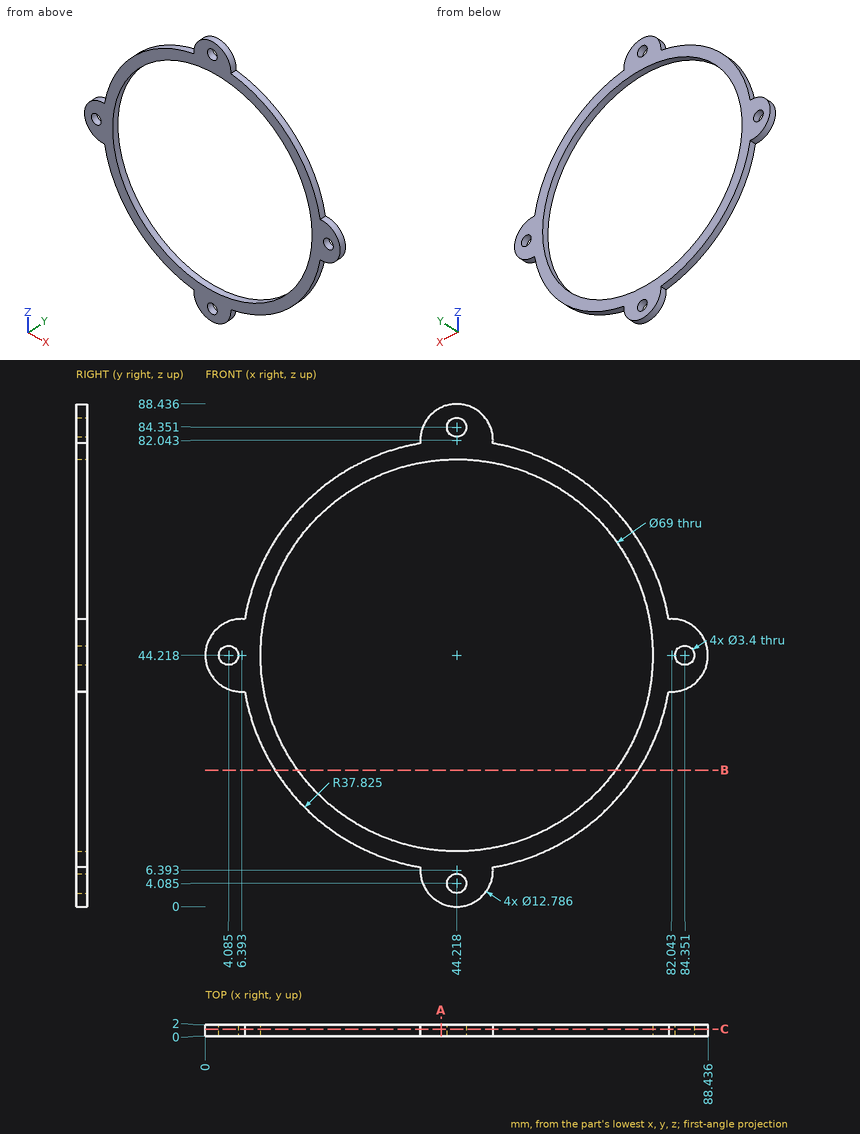
Design review of the part shown in the three views and the two pictorial views. Dimensions are in mm from the part's minimum x, y and z. Round coordinates to 2 decimals unless told otherwise and drop trailing zeros. Loops run counter-clockwise (first coordinate to the right, second up) from the corner with the lowest first, then second, coordinate; pieces in that order, holes last. Notation, with made-up numbers: M -2.5,-29.75 L 24.5,-29.75 A16 ccw 24.5,-4.75 Z; hole C 3.25,58 d11. An arc over 180 degrees is marked long. Answer as a JSON object with one key per item and string values.
Item 1: We need section A-A, the plane x = 41.5. State the section outline as (y, z) points (1 decimal).
Check sheet entries:
{"outline": "M 0,0.6 L 2,0.6 L 2,9.8 L 0,9.8 Z; M 0,78.6 L 2,78.6 L 2,87.8 L 0,87.8 Z"}
Item 2: We need section B-B, the plane z = 24. State the section outline as (x, y) points.
Check sheet entries:
{"outline": "M 12.25,0 L 16.26,0 L 16.26,2 L 12.25,2 Z; M 72.17,0 L 76.19,0 L 76.19,2 L 72.17,2 Z"}
Item 3: For line 1 along X through (y, z) = (1.6, 68.5) (1 decimal); line 2 along Z through (x, y) = (53, 0.85) (1 decimal); line 3 along Z through (x, y) = (34, 0.9), list the stretches that pass through material, from the lowest coordinate up.
Check sheet entries:
{"line 1": "15.2 to 19.7, 68.7 to 73.2", "line 2": "7.4 to 10.9, 77.6 to 81", "line 3": "7.8 to 11.27, 77.17 to 80.64"}
Item 4: We need section C-C, the plane y = 1.2. State how many separate pieces and enclosed holes the cut face has, and give its area (3 significant figures).
Check sheet entries:
{"separate pieces": "1", "enclosed holes": "5", "area": "985 mm2"}
